from build123d import *

# Parameters (mm, degrees)
BASE_FLANGE1_DEPTH      = 550
SKETCH10_R              = 3
CUT_EXTRUDE2_DEPTH      = 10
CUT_EXTRUDE3_DEPTH      = 587.003412959
CUT_EXTRUDE3_DEPTH_BACK = 587.003412959
SKETCH15_W              = 2
SKETCH15_H              = 199.2634
BOSS_EXTRUDE2_DEPTH     = 50
SKETCH16_W              = 32
SKETCH16_H              = 2
CUT_EXTRUDE4_DEPTH      = 2.7366


# Sheet-metal steps are written as plain solids
with BuildPart() as part:
    # Sketch1 → Base-Flange1 (new body)
    with BuildSketch(Plane.XY):
        with BuildLine():
            Line((0, 0), (29.2634, 0))
            ThreePointArc((29.2634, 0), (29.784254855, 0.215745145), (30, 0.7366))
            Line((30, 0.7366), (30, 200))
            Line((30, 200), (32, 200))
            Line((32, 200), (32, 0.7366))
            ThreePointArc((32, 0.7366), (31.198468417, -1.198468417), (29.2634, -2))
            Line((29.2634, -2), (0, -2))
            Line((0, -2), (0, 0))
        make_face()
    extrude(amount=BASE_FLANGE1_DEPTH)

    # Sketch10 → Cut-Extrude2 (cut)
    with BuildSketch(Plane(origin=(32, 0, 0), x_dir=(0, 0, -1), z_dir=(1, 0, 0))):
        with Locations((-500, 58)):
            Circle(SKETCH10_R)
        with Locations((-440, 58)):
            Circle(SKETCH10_R)
        with Locations((-380, 58)):
            Circle(SKETCH10_R)
        with Locations((-320, 58)):
            Circle(SKETCH10_R)
        with Locations((-260, 58)):
            Circle(SKETCH10_R)
        with Locations((-200, 58)):
            Circle(SKETCH10_R)
        with Locations((-140, 58)):
            Circle(SKETCH10_R)
    extrude(amount=-CUT_EXTRUDE2_DEPTH, mode=Mode.SUBTRACT)

    # Sketch11 → Cut-Extrude3 (cut, two sides: drawn at the far end of the back side and taken through both)
    with BuildSketch(Plane.ZY.offset(-30).offset(-CUT_EXTRUDE3_DEPTH_BACK)):
        Polygon((0, 200), (95, 200), (95, 0.7366), (95, -11.499359117), (0, -11.499359117), (0, 0.7366), align=None)
    extrude(amount=CUT_EXTRUDE3_DEPTH + CUT_EXTRUDE3_DEPTH_BACK, mode=Mode.SUBTRACT)

    # Sketch15 → Boss-Extrude2 (add)
    with BuildSketch(Plane(origin=(32, 0, 0), x_dir=(0, 0, -1), z_dir=(1, 0, 0))):
        with Locations((-96, 100.3683)):
            Rectangle(SKETCH15_W, SKETCH15_H)
    extrude(amount=BOSS_EXTRUDE2_DEPTH)

    # Sketch16 → Cut-Extrude4 (cut)
    with BuildSketch(Plane(origin=(0, -2, 0), x_dir=(-1, 0, 0), z_dir=(0, -1, 0))):
        with Locations((-16, -96)):
            Rectangle(SKETCH16_W, SKETCH16_H)
    extrude(amount=-CUT_EXTRUDE4_DEPTH, mode=Mode.SUBTRACT)


solid = part.part
For this review, take the finished solid that the model builds, in its own axes (mm). A direction names the side the tool comes from. Round coordinates to 2 decimals unless told otherwise and drop trailing zeros. Order: outer loops, then holes, each group sorted by start corner. A loop starts at its lowest first (then second) coordinate and runs counter-clockwise, first axis right, second up. Notation, with made-up numbers: (66.25, -31.75) -> (110.25, -31.75) arc R22 cw to (110.25, -11.75) -> close; hole circle Ø7 at (33.5, -11.75). An arc over 180 degrees is marked (long way). Put each result on its own line as item: value.
Q1. Add section B-B on y = 185. Write out the cut boundary in (x, z), plus the area to 3 significant figures.
Check result:
outline: (30, 95) -> (82, 95) -> (82, 97) -> (32, 97) -> (32, 550) -> (30, 550) -> close
area: 1,010 mm2
Q2. For probe 1 along X at (y, z) = (21, 378.5); probe 2 along Z at (x, y) = (50.5, 175.5); probe 3 along Y at (x, z) = (31, 140), list the stretches that pass through material, from the lowest coordinate up. Write a range as [from, to].
Check result:
probe 1: [30, 32]
probe 2: [95, 97]
probe 3: [-1.38, 55], [61, 200]
Q3. Add section A-A on x = 49. Write out the cut boundary in (y, z), plus the area to 3 significant figures.
Check result:
outline: (0.74, 95) -> (200, 95) -> (200, 97) -> (0.74, 97) -> close
area: 399 mm2
Q4. Insertion check: pin 1 Ø1.6 at (x, z) = (63.5, 96) entering from -Y; pin 2 Ø8 at (y, z) = (58, 260) entering from -X; pin 3 Ø3 at (y, z) = (63.5, 143.5) entering from +X. Each pin has a flat end and moves straight along its axis. Give the tip position at first contact, or say it passes through.
Check result:
pin 1: y = 0.74
pin 2: x = 30
pin 3: x = 32
Q5. Machinability: for faces 1 (the flat face through (32, 102, 320)), 2 (the flat face through (56, 99, 95)), 3 (the flat face through (30, 99, 319)), which of the approach directions +Z, -Z, +X, -X, +Y, -Y give a long, thin tool a straight path to every point of the face, cutting with its end or side? Answer none if there is none.
Check result:
face 1: +Z, +X, +Y, -Y
face 2: -Z, +X, -X, +Y, -Y
face 3: +Z, -Z, -X, +Y
